For this review, use the dimensioned drawing (mm, ordinates from the lowest corner) and the shaded views. Coordinates: 2 decimals unless noted, no trailing zeros. Order: outer loops, then holes, each group sorted by start corner. A loop starts at its lowest first (then second) coordinate and runs counter-clockwise, first axis right, second up. Notation, with made-up numbers: M 71.25,-26 L 124.25,-26 A12 cw 124.25,-4 Z; hole C -26.75,64.5 d1. An arc over 180 degrees is marked long. One line per item, written item: value.
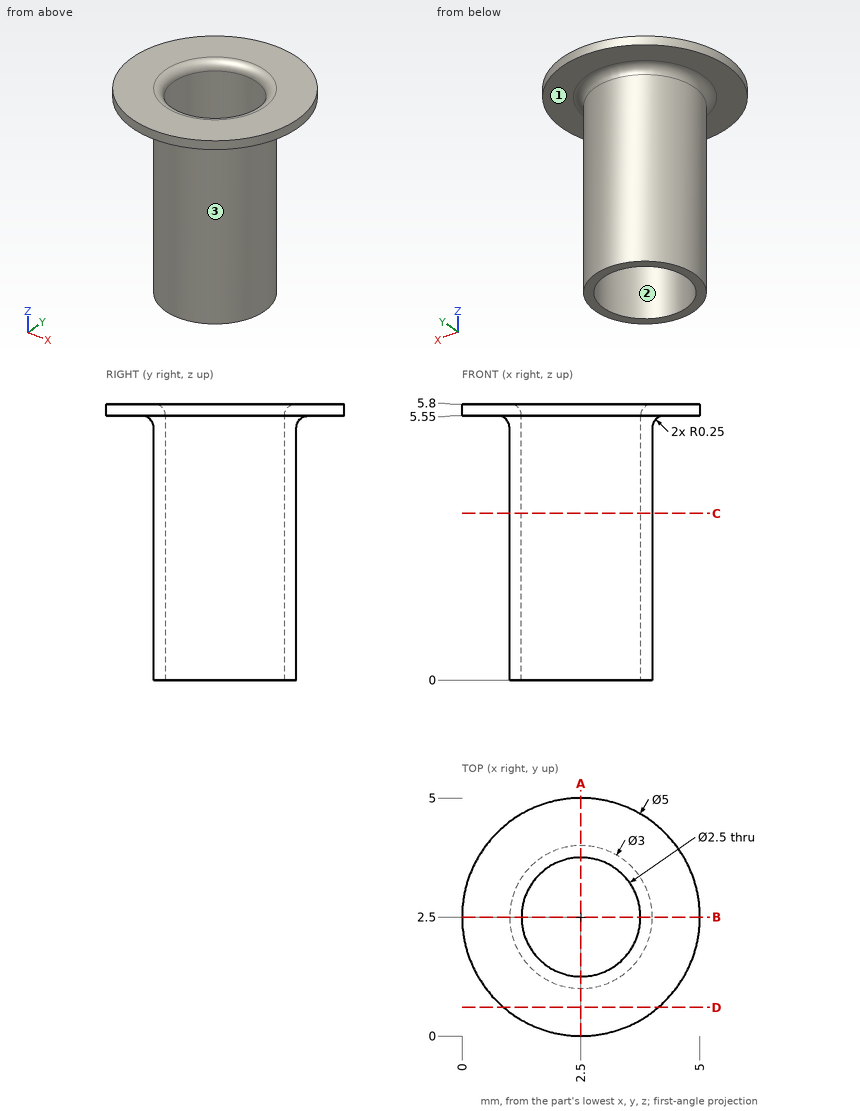
(1) Insertion check: pin 1 Ø1 at (x, z) = (4, 4) entering from -Y; pin 2 Ø1 at (y, z) = (4, 4.5) entering from -X; pin 3 Ø3 at (y, z) = (1, 3) entering from +X. Each pin has a flat end and moves straight along its axis. Give the tip position at first contact, or say it passes through.
Geometry results:
pin 1: stops at y = 1.38
pin 2: stops at x = 1.38
pin 3: stops at x = 4
(2) We need section D-D, the plane y = 0.6. State the section outline as (x, z) points.
Geometry results:
outline: M 0.88,5.55 L 4.12,5.55 L 4.12,5.8 L 0.88,5.8 Z
(3) We need section A-A, the plane x = 2.5. State the section outline as (y, z) points.
Geometry results:
outline: M 0,5.55 L 0.75,5.55 A0.25 cw 1,5.3 L 1,0 L 1.25,0 L 1.25,5.55 A0.25 ccw 1,5.8 L 0,5.8 Z; M 3.75,0 L 4,0 L 4,5.3 A0.25 cw 4.25,5.55 L 5,5.55 L 5,5.8 L 4,5.8 A0.25 ccw 3.75,5.55 Z
(4) For L1, parallel to Y at x = 2.5, z = 1.55; L2, parallel to Z at x = 0.5, y = 2.95; L3, parallel to X at y = 2.25, z = 3.4, list the stretches that pass through material, from the lowest coordinate up.
Geometry results:
L1: y = 1 to 1.25, 3.75 to 4
L2: z = 5.55 to 5.8
L3: x = 1.02 to 1.28, 3.72 to 3.98
(5) Mouldability with a two-part tool opening along X and no side actions: class the marked faces 1, 2 and 3 as +X half, -X half, draft (parallel to the pull), parting line (faces both ways), or undercut.
Geometry results:
face 1: draft
face 2: undercut
face 3: parting line
(6) We need section C-C, the plane z = 3.5. State the section outline as (x, y) points, plus the area to 3 significant figures.
Geometry results:
outline: C 2.5,2.5 d3; hole C 2.5,2.5 d2.5
area: 2.16 mm2
